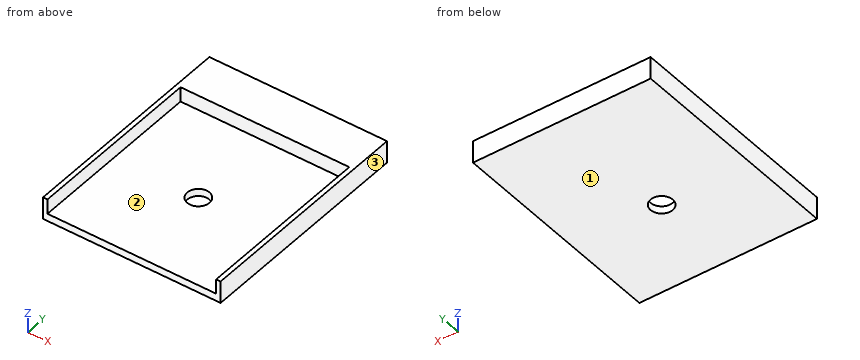
from build123d import *

# Parameters (mm, degrees)
SKETCH1_W           = 120
SKETCH1_H           = 150
BOSS_EXTRUDE1_DEPTH = 5
BOSS_EXTRUDE2_DEPTH = 10
SKETCH4_R           = 7.5
CUT_EXTRUDE1_DEPTH  = 10


with BuildPart() as part:
    # Sketch1 → Boss-Extrude1 (new body)
    with BuildSketch(Plane.XY):
        Rectangle(SKETCH1_W, SKETCH1_H)
    extrude(amount=BOSS_EXTRUDE1_DEPTH)

    # Sketch3 → Boss-Extrude2 (add)
    with BuildSketch(Plane.XY.offset(5)):
        Polygon((-60, 45), (-60, -75), (-57, -75), (-57, 45), (57, 45), (57, -75), (60, -75), (60, 45), (60, 75), (-60, 75), align=None)
    extrude(amount=BOSS_EXTRUDE2_DEPTH)

    # Sketch4 → Cut-Extrude1 (cut)
    with BuildSketch(Plane(origin=(0, 0, 0), x_dir=(-1, 0, 0), z_dir=(0, 0, -1))):
        with Locations((0, -15)):
            Circle(SKETCH4_R)
    extrude(amount=-CUT_EXTRUDE1_DEPTH, mode=Mode.SUBTRACT)


solid = part.part
Input: part model. Units: mm. Frame: model coordinates. Face numbers are marked on the shaded views. Round coordinates to 2 decimals unless told otherwise and drop trailing zeros. Order: outer loops, then holes, each group sorted by start corner. A loop starts at its lowest first (then second) coordinate and runs counter-clockwise, first axis right, second up.
1. Mould query, pull axis X, two halves, no side actions, for the marked faces 1, 2 and 3. Classes: released by +X, released by -X, zero draft, split by the parting line, or undercut.
The answers:
face 1: zero draft
face 2: undercut
face 3: released by +X
2. Pin query (flat end, axial travel): P1, Ø1, axis at x = 10.5, z = 7.5, coming from the -Y side; P2, Ø10, axis at x = -46.5, y = -20.5, coming from the -Z side; P3, Ø2, axis at x = -8.5, y = -33, coming from the +Z side. Return the tip coordinate at first contact, or that it passes through.
The answers:
P1: stops at y = 45
P2: stops at z = 0
P3: stops at z = 5
3. Cut plane B-B, the plane y = -15. Output: boundary loops of the cut face in (x, z), then the cut area to 3 significant figures.
The answers:
outline: (-60, 0) - (-7.5, 0) - (-7.5, 5) - (-57, 5) - (-57, 15) - (-60, 15) - close; (7.5, 0) - (60, 0) - (60, 15) - (57, 15) - (57, 5) - (7.5, 5) - close
area: 585 mm2
4. Material intervals for line 1 (Y direction, x = 0, z = 2.05); line 2 (X direction, y = 0, z = 13.25); line 3 (Y direction, x = -25, z = 13.75), sorted ascending.
The answers:
line 1: y = -75 to -22.5, -7.5 to 75
line 2: x = -60 to -57, 57 to 60
line 3: y = 45 to 75
5. Cut plane C-C, the plane z = 10. Output: boundary loops of the cut face in (x, y).
The answers:
outline: (-60, -75) - (-57, -75) - (-57, 45) - (57, 45) - (57, -75) - (60, -75) - (60, 75) - (-60, 75) - close
6. Cut plane D-D, the plane x = -18.5. Output: boundary loops of the cut face in (y, z).
The answers:
outline: (-75, 0) - (75, 0) - (75, 15) - (45, 15) - (45, 5) - (-75, 5) - close
7. Cut plane A-A, the plane x = 0. Output: boundary loops of the cut face in (y, z).
The answers:
outline: (-75, 0) - (-22.5, 0) - (-22.5, 5) - (-75, 5) - close; (-7.5, 0) - (75, 0) - (75, 15) - (45, 15) - (45, 5) - (-7.5, 5) - close
